Read the model definition and answer for the solid it produces. Units are mm, in the model's axes. A direction names the side the tool comes from. Coordinates: 2 decimals unless noted, no trailing zeros. Loops run counter-clockwise (first coordinate to the right, second up) from the corner with the lowest first, then second, coordinate; pieces in that order, holes last. Notation, with made-up numbers: (-34.75, -25.75) - (-14.75, -25.75) arc R23 ccw to (-14.75, 1.25) - close; hole circle Ø5 at (0.5, 44.25). An arc over 180 degrees is marked (long way). Use one line per item in the form item = value. Start each with the question number.
1) Consider line 1 (X direction, y = 13, z = 0); line 2 (Z direction, x = -18, y = 7); line 3 (X direction, y = 12, z = -22). Determine where each line is inside the solid, lowest interval first.
2) Each of these flat-tipped pins is pushed along its axis until it touches: P1, Ø3.5, axis at x = -9.06, z = -17.27, coming from the -Y side; P2, Ø5, axis at y = 15.5, z = 11.5, coming from the +X side; P3, Ø1.1, axis at y = 10, z = 5, coming from the +X side; P4, Ø3, axis at x = 12, y = 7, coming from the +Z side. Where does it stop, or does it pass through?
3) The mould has two halves that part along X. Classify faces 1 (the face through (16.3, 9.86, -18.29)), 2 (the face through (14.61, 10.14, 17.62)), 3 (the face through (-0.1, 9.9, 24.5)), 4 (the face through (0.75, 10, -23)): released by +X, released by -X, zero draft, split by the parting line, or undercut.
4) Which of the six approach directions +Z, -Z, +X, -X, +Y, -Y give full straight-line access (tool end or side, diameter ignored) to faces 5 (the face through (0, 0, 5)), 6 (the face through (-15.734, 10.14, 16.629))?
5) A cutting plane is placed at A-A (x = 0). Give the vertices of the cut face in (y, z), and give its area (3 significant figures).
6) A cutting plane is placed at B-B (z = -20.5). Give the vertices of the cut face in (x, y), and give its area (3 significant figures).
7) A cutting plane is placed at C-C (x = 7.5). Give the vertices of the cut face in (y, z), and give its area (3 significant figures).
from build123d import *

# Parameters (mm, degrees)
SKETCH1_R                = 24.5
BOSS_EXTRUDE1_DEPTH      = 20
CUT_EXTRUDE1_DEPTH       = 41.006249512
FILLET1_R                = 0.25
CIRPATTERN1_COUNT        = 13
FILLET1_OF_CIRPATTERN1_R = 0.25


with BuildPart() as part:
    # Sketch1 → Boss-Extrude1 (new body)
    with BuildSketch(Plane(origin=(0, 0, 0), x_dir=(1, 0, 0), z_dir=(0, 1, 0))):
        with Locations(Location((0, 0, 0), (0, 0, 270))):
            Circle(SKETCH1_R)
        with BuildLine():
            Line((2, -5.667459748), (2, -3.51))
            Line((2, -3.51), (-2, -3.51))
            Line((-2, -3.51), (-2, -5.667459748))
            ThreePointArc((-2, -5.667459748), (0, 6.01), (2, -5.667459748))
        make_face(mode=Mode.SUBTRACT)
    extrude(amount=BOSS_EXTRUDE1_DEPTH)

    # Sketch3 → Cut-Extrude1 (cut, through all)
    with BuildSketch(Plane(origin=(0, 20, 0), x_dir=(1, 0, 0), z_dir=(0, 1, 0))):
        with BuildLine():
            Line((0.75, 21.568211788), (0.75, 24.5))
            Line((0.75, 24.5), (-0.75, 24.5))
            Line((-0.75, 24.5), (-0.75, 21.568211788))
            ThreePointArc((-0.75, 21.568211788), (0, 17.3), (0.75, 21.568211788))
        make_face()
    cut_extrude1 = extrude(amount=-CUT_EXTRUDE1_DEPTH, mode=Mode.SUBTRACT)

    # Fillet1
    fillet1_edges = [part.edges().sort_by_distance(p)[0] for p in [
        (0.75, 10, -24.488517717),
        (-0.75, 10, -24.488517717),
    ]]
    fillet(fillet1_edges, radius=FILLET1_R)

    # CirPattern1: Cut-Extrude1 ×13 about axis
    cirpattern1_axis = Axis((0, 0, 0), (0, 1, 0))
    for i in range(1, CIRPATTERN1_COUNT):
        add(cut_extrude1.rotate(cirpattern1_axis, i * 360 / CIRPATTERN1_COUNT), mode=Mode.SUBTRACT)

    # Fillet1 of CirPattern1
    fillet1_of_cirpattern1_edges = [part.edges().sort_by_distance(p)[0] for p in [
        (-10.716289613, 10, -22.032047951),
        (-12.044473652, 10, -21.334963193),
        (-19.727606421, 10, -14.528301514),
        (-20.579703541, 10, -13.293825716),
        (-24.219566341, 10, -3.696296286),
        (-24.400371362, 10, -2.207232974),
        (-23.16311549, 10, 7.982485877),
        (-22.63120816, 10, 9.385010241),
        (-16.800274026, 10, 17.832576725),
        (-15.677507904, 10, 18.827260712),
        (-6.588692248, 10, 23.59743915),
        (-5.132279522, 10, 23.956412647),
        (5.132279522, 10, 23.956412647),
        (6.588692248, 10, 23.59743915),
        (15.677507904, 10, 18.827260712),
        (16.800274026, 10, 17.832576725),
        (22.63120816, 10, 9.385010241),
        (23.16311549, 10, 7.982485877),
        (24.400371362, 10, -2.207232974),
        (24.219566341, 10, -3.696296286),
        (20.579703541, 10, -13.293825716),
        (19.727606421, 10, -14.528301514),
        (12.044473652, 10, -21.334963193),
        (10.716289613, 10, -22.032047951),
    ]]
    fillet(fillet1_of_cirpattern1_edges, radius=FILLET1_OF_CIRPATTERN1_R)


solid = part.part
Found:
q1.line_1 = -24.5 to -6.01, 6.01 to 24.5
q1.line_2 = -16.62 to -13.34, -10.06 to -4.08, -0.62 to 4.73, 9.1 to 16.62
q1.line_3 = -10.61 to -0.75, 0.75 to 10.61
q2.P1 = through
q2.P2 = 22.55
q2.P3 = 24.09
q2.P4 = 22.14
q3.face_1 = released by +X
q3.face_2 = undercut
q3.face_3 = split by the parting line
q3.face_4 = undercut
q4.face_5 = +Z, -Z, +X, -X, -Y
q4.face_6 = +Y, -Y
q5.outline = (0, -17.3) - (20, -17.3) - (20, -6.01) - (0, -6.01) - close; (0, 3.51) - (20, 3.51) - (20, 24.5) - (0, 24.5) - close
q5.area = 646 mm^2
q6.outline = (-13.42, 0) - (-11.61, 0) - (-11.61, 20) - (-13.42, 20) - close; (-9.91, 0) - (-1.96, 0) - (-1.96, 20) - (-9.91, 20) - close; (1.96, 0) - (9.91, 0) - (9.91, 20) - (1.96, 20) - close; (11.61, 0) - (13.42, 0) - (13.42, 20) - (11.61, 20) - close
q6.area = 391 mm^2
q7.outline = (0, -23.32) - (20, -23.32) - (20, -18.82) - (0, -18.82) - close; (0, -15.72) - (20, -15.72) - (20, 23.32) - (0, 23.32) - close
q7.area = 871 mm^2
